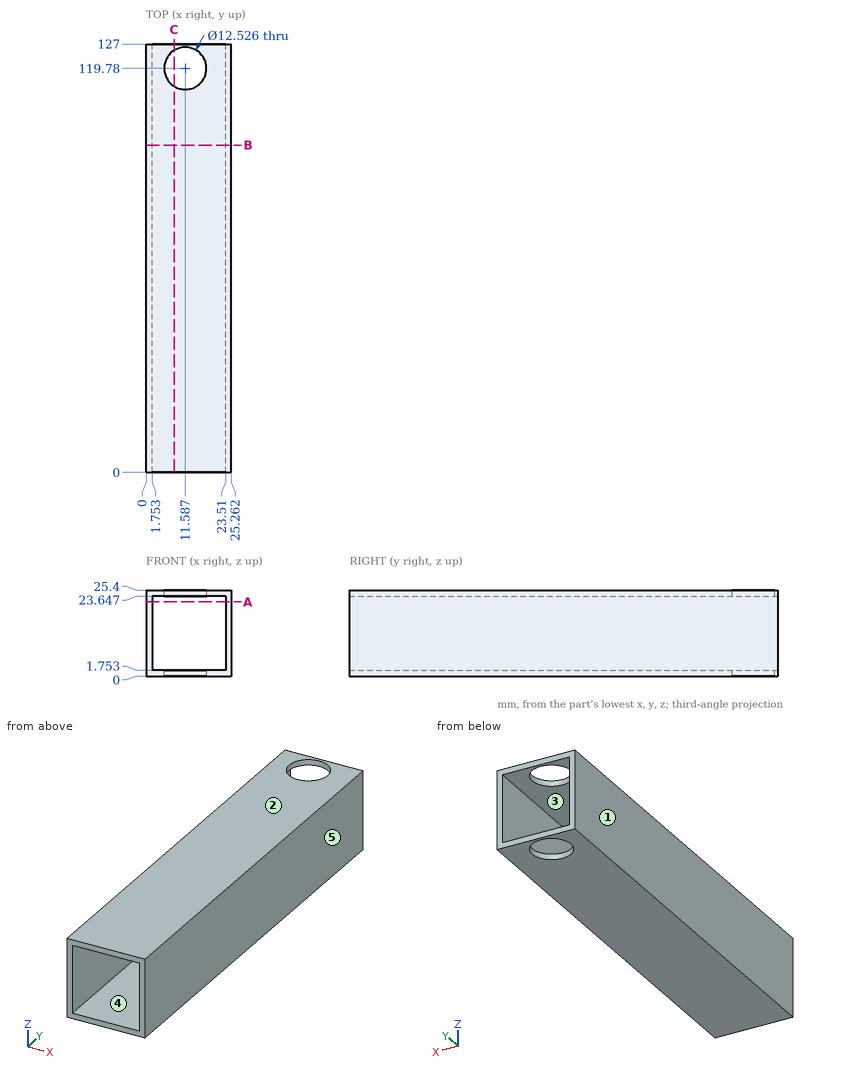
Verification items for this drawing (mm, ordinates from the low corner). A direction names the side the tool comes from. Coordinates: 2 decimals unless noted, no trailing zeros. Loops run counter-clockwise (first coordinate to the right, second up) from the corner with the lowest first, then second, coordinate; pieces in that order, holes last. Notation, with made-up numbers: (48, -19.5) - (98, -19.5) arc R14 cw to (98, -15.5) - close; hole circle Ø3 at (9.25, 31.25). An arc over 180 degrees is marked (long way). Use one line per item in the form item = value. Start each with the question number.
Item 1: Mould release check, pull along Z, two halves, no side actions. Record for the marked faces 1, 2 and 3: +Z half, -Z half, draft (parallel to the pull), parting line (faces both ways), or undercut.
Item 2: Section check A-A, the plane z = 22. Enter the section's corners in (x, y).
Item 3: Section check B-B, the plane y = 97. Enter the section's corners in (x, z).
Item 4: Section check C-C, the plane x = 8.25. Enter the section's corners in (y, z), and give its area (3 significant figures).
Item 5: Gauge pin test, flat end, axial feed: pin 1 (10 mm diameter, centred on x = 9, y = 14, fed in from -Z). Record the tip position at first contact, or that the pin passes through.
Item 6: Thickness scan on probe 1 along X at (y, z) = (25.5, 4.25); probe 2 along Z at (x, y) = (15.75, 104). Record the ranges inside material, lowest first.
Item 7: Tool access check on the marked faces 4 and 5. Record the directions out of +Z, -Z, +X, -X, +Y, -Y that give a thin tool (end or side, any length) a straight path to the whole face; none if there is none.
Computed:
q1.face_1 = draft
q1.face_2 = +Z half
q1.face_3 = undercut
q2.outline = (0, 0) - (1.75, 0) - (1.75, 127) - (0, 127) - close; (23.51, 0) - (25.26, 0) - (25.26, 127) - (23.51, 127) - close
q3.outline = (0, 0) - (25.26, 0) - (25.26, 25.4) - (0, 25.4) - close; hole (1.75, 1.75) - (23.51, 1.75) - (23.51, 23.65) - (1.75, 23.65) - close
q4.outline = (0, 0) - (114.48, 0) - (114.48, 1.75) - (0, 1.75) - close; (0, 23.65) - (114.48, 23.65) - (114.48, 25.4) - (0, 25.4) - close; (125.08, 0) - (127, 0) - (127, 1.75) - (125.08, 1.75) - close; (125.08, 23.65) - (127, 23.65) - (127, 25.4) - (125.08, 25.4) - close
q4.area = 408 mm2
q5.pin_1 = 0
q6.probe_1 = 0 to 1.75, 23.51 to 25.26
q6.probe_2 = 0 to 1.75, 23.65 to 25.4
q7.face_4 = +Y, -Y
q7.face_5 = +Z, -Z, +X, +Y, -Y
